```python
from build123d import *

# Parameters (mm, degrees)
SALIENTE_EXTRUIR1_DEPTH   = 38
SALIENTE_EXTRUIR1_2_DEPTH = 38
CROQUIS2_R                = 1.5
SALIENTE_EXTRUIR2_DEPTH   = 2
SALIENTE_EXTRUIR4_DEPTH   = 17
CROQUIS4_R                = 4
CORTAR_EXTRUIR2_DEPTH     = 17


with BuildPart() as part:
    # Croquis1 → Saliente-Extruir1 (new body)
    with BuildSketch(Plane.XY):
        with BuildLine():
            Line((10.5, 0), (10.5, 10.5))
            Line((10.5, 10.5), (10.5, 17))
            Line((10.5, 17), (2.5, 17))
            Line((2.5, 17), (2.5, 10.198039027))
            ThreePointArc((2.5, 10.198039027), (8.261355821, 6.480740698), (10.5, 0))
        make_face()
    extrude(amount=SALIENTE_EXTRUIR1_DEPTH)



with BuildPart() as body_2:
    # Croquis1 → Saliente-Extruir1 2 (new body)
    with BuildSketch(Plane.XY):
        with BuildLine():
            Line((-10.5, 0), (-10.5, 10.5))
            Line((-10.5, 10.5), (-10.5, 17))
            Line((-10.5, 17), (-2.5, 17))
            Line((-2.5, 17), (-2.5, 10.198039027))
            ThreePointArc((-2.5, 10.198039027), (-8.261355821, 6.480740698), (-10.5, 0))
        make_face()
    extrude(amount=SALIENTE_EXTRUIR1_2_DEPTH)


with BuildPart() as part_1:
    add(part.part)

    add(body_2.part)  # Saliente-Extruir2 merges body 2
    # Croquis2 → Saliente-Extruir2 (add)
    with BuildSketch(Plane(origin=(0, 17, 0), x_dir=(1, 0, 0), z_dir=(0, 1, 0))):
        Polygon((2.5, 0), (-2.5, 0), (-2.5, -40), (-12.5, -40), (-17.5, -40), (-17.5, 2), (-17.5, 3), (17.5, 3), (17.5, 2), (17.5, -40), (12.5, -40), (2.5, -40), align=None)
        with Locations((-15, -3)):
            Circle(CROQUIS2_R, mode=Mode.SUBTRACT)
        with Locations((15, -3)):
            Circle(CROQUIS2_R, mode=Mode.SUBTRACT)
        with Locations((15, -35)):
            Circle(CROQUIS2_R, mode=Mode.SUBTRACT)
        with Locations((-15, -35)):
            Circle(CROQUIS2_R, mode=Mode.SUBTRACT)
    extrude(amount=-SALIENTE_EXTRUIR2_DEPTH)

    # Croquis3 → Saliente-Extruir4 (add)
    with BuildSketch(Plane(origin=(0, 17, 0), x_dir=(1, 0, 0), z_dir=(0, 1, 0))):
        Polygon((0, 3), (-4, 3), (-4, 0), (3.996992923, 0), (3.996992923, 3), align=None)
    extrude(amount=-SALIENTE_EXTRUIR4_DEPTH)

    # Croquis4 → Cortar-Extruir2 (cut)
    with BuildSketch(Plane(origin=(0, 0, -3), x_dir=(-1, 0, 0), z_dir=(0, 0, -1))):
        Circle(CROQUIS4_R)
    extrude(amount=-CORTAR_EXTRUIR2_DEPTH, mode=Mode.SUBTRACT)


solid = part_1.part
```
For this review, take the finished solid that the model builds, in its own axes (mm). A direction names the side the tool comes from. Round coordinates to 2 decimals unless told otherwise and drop trailing zeros. Order: outer loops, then holes, each group sorted by start corner. A loop starts at its lowest first (then second) coordinate and runs counter-clockwise, first axis right, second up.
Q1. Machinability: for faces 4 (the flat face through (-4, 8, -2)), 5 (the flat face through (10.5, 7, 19)), 6 (the flat face through (3.997, 8, -1)), 7 (the flat face through (2.5, 14, 20)), which of the approach directions +Z, -Z, +X, -X, +Y, -Y give a long, thin tool a straight path to every point of the face, cutting with its end or side? Answer none if there is none.
Findings below:
face 4: -Z, -X, -Y
face 5: +Z, -Z, +X, -Y
face 6: -Z, +X, -Y
face 7: +Z, +Y, -Y
Q2. We need section C-C, the plane y = 7.5. Give the boundary of the cut face in (x, z).
Findings below:
outline: (-10.5, 0) - (-7.35, 0) - (-7.35, 38) - (-10.5, 38) - close; (-4, -3) - (4, -3) - (4, 0) - (-4, 0) - close; (7.35, 0) - (10.5, 0) - (10.5, 38) - (7.35, 38) - close
Q3. Wall thickness on line 1 (X direction, y = 16.5, z = 35); line 2 (Z direction, x = 15, y = 16.05); line 3 (X direction, y = 10.75, z = 22): over which ranges is each line inside the solid? List them lowest first.
Findings below:
line 1: x = -17.5 to -16.5, -13.5 to -2.5, 2.5 to 13.5, 16.5 to 17.5
line 2: z = -3 to 1.5, 4.5 to 33.5, 36.5 to 40
line 3: x = -10.5 to -2.5, 2.5 to 10.5
Q4. Insertion check: P1, Ø3, axis at x = -9.5, y = 7.5, coming from the -Z side; P2, Ø10, axis at y = 8.5, z = 24.5, coming from the +X side; P3, Ø6.5, axis at x = -7, y = 6.5, coming from the +Z side. Each pin has a flat end and moves straight along its axis. Give the tip position at first contact, or say it passes through.
Findings below:
P1: stops at z = 0
P2: stops at x = 10.5
P3: stops at z = 38
Q5. We need section D-D, the plane x = -5. Give the boundary of the cut face in (y, z), plus the area to 3 significant figures.
Findings below:
outline: (9.23, 0) - (15, 0) - (15, -3) - (17, -3) - (17, 40) - (15, 40) - (15, 38) - (9.23, 38) - close
area: 305 mm2
Q6. We need section B-B, the plane z = 7. Give the boundary of the cut face in (x, y), plus the area to 3 significant figures.
Findings below:
outline: (-17.5, 15) - (-10.5, 15) - (-10.5, 0) arc R10.5 cw to (-2.5, 10.2) - (-2.5, 17) - (-17.5, 17) - close; (2.5, 10.2) arc R10.5 cw to (10.5, 0) - (10.5, 15) - (17.5, 15) - (17.5, 17) - (2.5, 17) - close
area: 179 mm2
Q7. We need section A-A, the plane x = 15. Give the boundary of the cut face in (y, z).
Findings below:
outline: (15, -3) - (17, -3) - (17, 1.5) - (15, 1.5) - close; (15, 4.5) - (17, 4.5) - (17, 33.5) - (15, 33.5) - close; (15, 36.5) - (17, 36.5) - (17, 40) - (15, 40) - close
Q8. Mouldability with a two-part tool opening along Z and no side actions: class faces 1 (the cylindrical face through (13.5, 16.01, 2.93)), 2 (the flat face through (0, 12, -3)), 3 (the flat face through (-10, 16, 40)) as pulls with the +Z half, pulls with the -Z half, needs draft (parallel to the pull), parting line crosses it, or undercut.
Findings below:
face 1: undercut
face 2: pulls with the -Z half
face 3: pulls with the +Z half
